Here's the drawing with two shaded views (mm, measured from the low corner). I have some questions. Round coordinates to 2 decimals unless told otherwise and drop trailing zeros. Order: outer loops, then holes, each group sorted by start corner. A loop starts at its lowest first (then second) coordinate and runs counter-clockwise, first axis right, second up. Notation, with made-up numbers: (-33.5, 26.5) -> (9.5, 26.5) arc R21 ccw to (9.5, 41.5) -> close; hole circle Ø7 at (5.25, -36.75). An arc over 180 degrees is marked (long way). Answer in a Markdown table with one row per item.
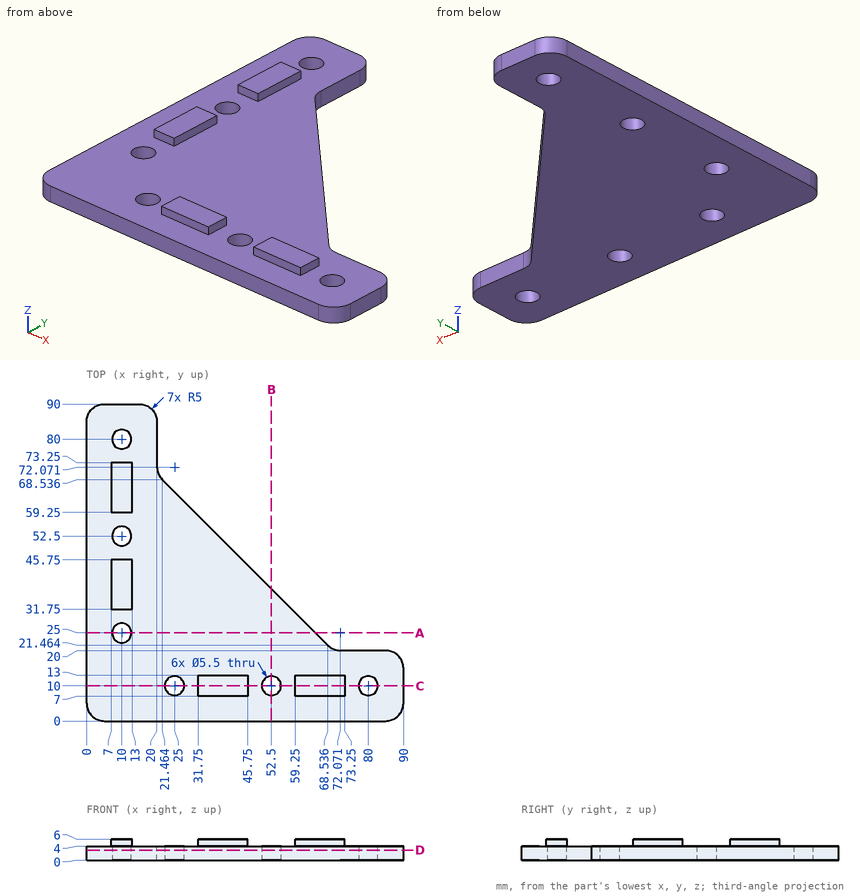
1. For pin 1 Ø1.6 at (x, z) = (9.5, 5.5) entering from +Y; pin 2 Ø1.6 at (x, z) = (63, 5) entering from +Y; pin 3 Ø0.6 at (y, z) = (11, 5.5) entering from +X, each with a flat end and sliding along its axis, tell me the tip position at first contact or that it passes through.
Numbers:
| item | result |
|---|---|
| pin 1 | stops at y = 73.25 |
| pin 2 | stops at y = 13 |
| pin 3 | stops at x = 73.25 |
2. Suppose I cut it at C-C on y = 10. Write out the boundary of the cut face in (x, z), then the cut area to 3 significant figures.
Numbers:
| item | result |
|---|---|
| outline | (0, 0) -> (22.25, 0) -> (22.25, 4) -> (0, 4) -> close; (27.75, 0) -> (49.75, 0) -> (49.75, 4) -> (45.75, 4) -> (45.75, 6) -> (31.75, 6) -> (31.75, 4) -> (27.75, 4) -> close; (55.25, 0) -> (77.25, 0) -> (77.25, 4) -> (73.25, 4) -> (73.25, 6) -> (59.25, 6) -> (59.25, 4) -> (55.25, 4) -> close; (82.75, 0) -> (90, 0) -> (90, 4) -> (82.75, 4) -> close |
| area | 350 mm2 |
3. Suppose I cut it at D-D on z = 2.85. State how many separate pieces and enclosed holes the cut face has, then the cut area to 3 significant figures.
Numbers:
| item | result |
|---|---|
| separate pieces | 1 |
| enclosed holes | 6 |
| area | 4,280 mm2 |
4. Suppose I cut it at A-A on y = 25. Write out the boundary of the cut face in (x, z).
Numbers:
| item | result |
|---|---|
| outline | (0, 0) -> (7.25, 0) -> (7.25, 4) -> (0, 4) -> close; (12.75, 0) -> (65, 0) -> (65, 4) -> (12.75, 4) -> close |
5. Suppose I cut it at B-B on x = 52.5. Write out the boundary of the cut face in (y, z).
Numbers:
| item | result |
|---|---|
| outline | (0, 0) -> (7.25, 0) -> (7.25, 4) -> (0, 4) -> close; (12.75, 0) -> (37.5, 0) -> (37.5, 4) -> (12.75, 4) -> close |
6. Please list where these lines run through material, in increasing order: line 1 along Y through (x, z) = (10, 1.2); line 2 along Y through (x, z) = (80, 2.2); line 3 along Z through (x, y) = (32, 33).
Numbers:
| item | result |
|---|---|
| line 1 | y = 0 to 22.25, 27.75 to 49.75, 55.25 to 77.25, 82.75 to 90 |
| line 2 | y = 0 to 7.25, 12.75 to 20 |
| line 3 | z = 0 to 4 |
